Could you check a few things on this drawing? It's one solid part, dimensions in mm from its lowest x, y, z. Round coordinates to 2 decimals unless told otherwise and drop trailing zeros. Order: outer loops, then holes, each group sorted by start corner. A loop starts at its lowest first (then second) coordinate and runs counter-clockwise, first axis right, second up. Notation, with made-up numbers: (35.25, 75) - (63.25, 75) arc R28 cw to (63.25, 102) - close; hole circle Ø9 at (83, 23.5). An arc over 180 degrees is marked (long way). Use one line per item in the form item = value.
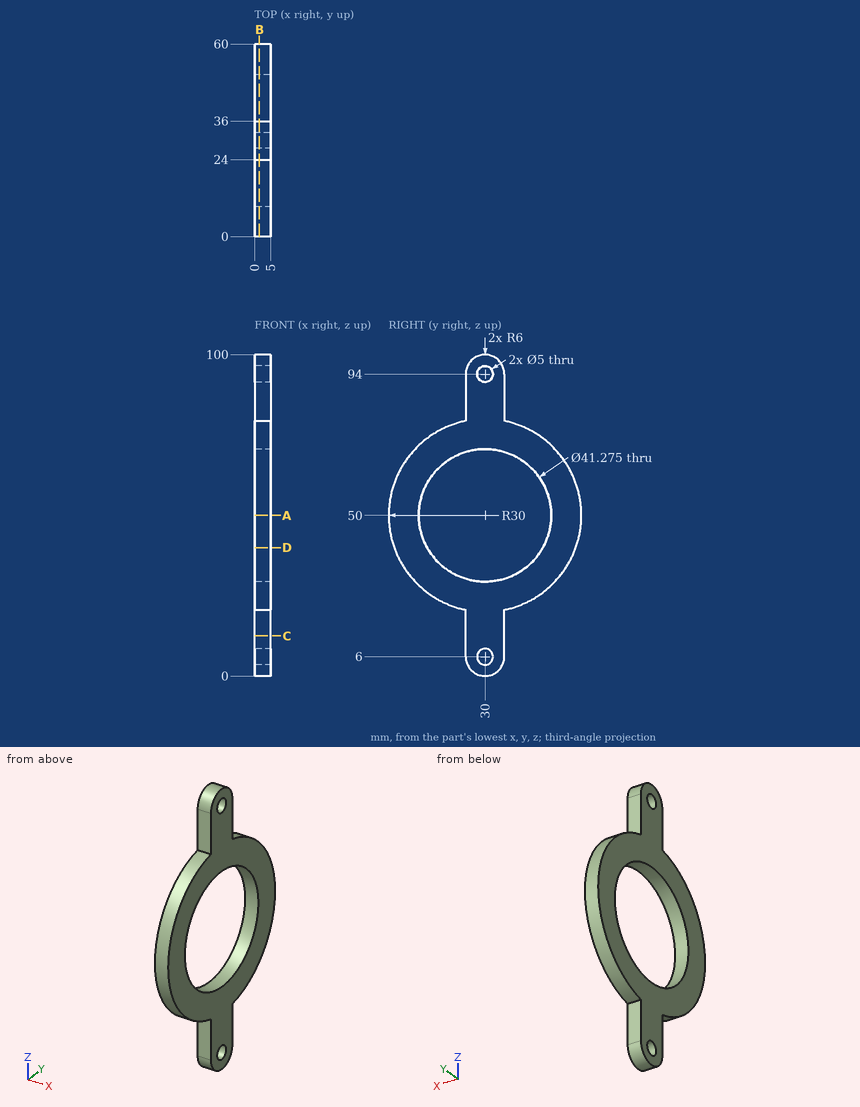
Item 1: Imagine slicing it at C-C on z = 12.5. Please give me the cut outline in (x, y).
Found:
outline = (0, 24) - (5, 24) - (5, 36) - (0, 36) - close
Item 2: I need wall thicknesses on L1, parallel to Y at x = 3.75, z = 94; L2, parallel to Z at x = 1.5, y = 35.5; L3, parallel to Z at x = 4.45, y = 28.5. Which ranges of each line are inside material? Lowest first, please.
Found:
L1 = 24 to 27.5, 32.5 to 36
L2 = 3.6 to 30.11, 69.89 to 96.4
L3 = 0.19 to 4, 8 to 29.42, 70.58 to 92, 96 to 99.81
Item 3: Will these pins go through, and if not, where does the flat tip stop? P1, Ø2, axis at x = 1.5, z = 39, coming from the +Y side; P2, Ø2.5, axis at x = 1.5, z = 12, coming from the +Y side; P3, Ø4.5, axis at y = 30, z = 6, coming from the -X side; P4, Ø1.5, axis at x = 3, z = 10.5, coming from the -Y side.
Found:
P1 = 58.28
P2 = 36
P3 = through
P4 = 24
Item 4: Imagine slicing it at B-B on x = 1.45. Please give me the cut outline in (y, z) (1 decimal), plus the area to 3 significant figures.
Found:
outline = (24, 6) arc R6 ccw to (36, 6) - (36, 20.6) arc R30 ccw to (36, 79.4) - (36, 94) arc R6 ccw to (24, 94) - (24, 79.4) arc R30 ccw to (24, 20.6) - close; hole circle Ø41.3 at (30, 50); hole circle Ø5 at (30, 6); hole circle Ø5 at (30, 94)
area = 1,900 mm2
Item 5: Imagine slicing it at A-A on z = 50. Please give me the cut outline in (x, y), plus the area to 3 significant figures.
Found:
outline = (0, 0) - (5, 0) - (5, 9.36) - (0, 9.36) - close; (0, 50.64) - (5, 50.64) - (5, 60) - (0, 60) - close
area = 93.6 mm2
Item 6: Imagine slicing it at D-D on z = 40. Please give me the cut outline in (x, y).
Found:
outline = (0, 1.72) - (5, 1.72) - (5, 11.95) - (0, 11.95) - close; (0, 48.05) - (5, 48.05) - (5, 58.28) - (0, 58.28) - close
